Work out the finished part from the listing and answer in its coordinate system (mm). A direction names the side the tool comes from. Coordinates: 2 decimals unless noted, no trailing zeros. Write each loop counter-clockwise with the first axis right and the second up, starting at its lowest first coordinate (ties: lowest second). Pieces come first, ordered by that corner, then holes. Notation, with made-up numbers: (-32.5, 57.5) - (21.5, 57.5) arc R10 ccw to (21.5, 73.5) - close; hole circle Ø11 at (4.25, -35). An arc over 180 degrees is marked (long way). Use a Markdown table: item, result. Add a question column.
(1) The part is cut by section D-D, the plane y = 15. Give the vertices of the cut face in (x, z).
(2) Find the intervals of material crossed by line 1 (Z direction, x = 32, y = 9.5); line 2 (X direction, y = 4.5, z = 38.05); line 3 (Y direction, x = 12.25, z = 2.25), in increasing order. Write a range as from..to.
(3) A tool of negligible diameter and unlimited length cuts with its end or side. For faces 1 (the face through (21.405, 20.021, 2.535)), 2 (the face through (20, 13, 5)), 3 (the face through (29.405, 20.021, 37.465)), from which of +Z, -Z, +X, -X, +Y, -Y can it reach the whole face along a straight path? Write none if from no direction.
(4) The part is cut by section A-A, the plane x = 16. Give the vertices of the cut face in (y, z), then the cut area to 3 significant figures.
(5) For a pull along Y with two mould halves and no side action, classify faces 4 (the face through (12.09, 13.74, 37.47)), 5 (the face through (20, 25, 20)), 6 (the face through (20, 12, 22.5)), 7 (the face through (29.405, 20.021, 2.535)) as released by +Y, released by -Y, zero draft, split by the parting line, or undercut.
(6) The part is cut by section B-B, the plane y = 11.75. State how many separate pieces and enclosed holes the cut face has, then the cut area to 3 significant figures.
(7) The part is cut by section C-C, the plane z = 27. Give the vertices of the cut face in (x, y).
(8) Given pin 1 Ø1.5 at (x, y) = (20.25, 4.5) entering from +Z; pin 2 Ø1 at (x, y) = (29, 5) entering from -Z; pin 3 Ø1.5 at (x, y) = (12.25, 4.5) entering from -Z, each flat-ended and moving along its own axis, determine where each tip first touches the part or whether it passes through.
from build123d import *

# Parameters (mm, degrees)
SKETCH1_W               = 40.5
SKETCH1_H               = 25
BOSS_EXTRUDE1_DEPTH     = 40
CUT_EXTRUDE1_START      = -5
SKETCH2_W               = 26.5
SKETCH2_H               = 25
CUT_EXTRUDE1_DEPTH      = 30
FILLET1_R               = 1
SKETCH3_R               = 1.25
CUT_EXTRUDE2_DEPTH      = 35
CUT_EXTRUDE2_DEPTH_BACK = 5
FILLET2_R               = 1
SKETCH6_W               = 5
SKETCH6_H               = 25
BOSS_EXTRUDE3_DEPTH     = 40.5


with BuildPart() as part:
    # Sketch1 → Boss-Extrude1 (new body)
    with BuildSketch(Plane.XY):
        with Locations((20.25, 12.5)):
            Rectangle(SKETCH1_W, SKETCH1_H)
    extrude(amount=BOSS_EXTRUDE1_DEPTH)

    # Sketch2 → Cut-Extrude1 (cut)
    with BuildSketch(Plane.XY.offset(40).offset(CUT_EXTRUDE1_START)):
        with Locations((20.25, 12.5)):
            Rectangle(SKETCH2_W, SKETCH2_H)
    extrude(amount=-CUT_EXTRUDE1_DEPTH, mode=Mode.SUBTRACT)

    # Fillet1
    fillet1_edges = [part.edges().sort_by_distance(p)[0] for p in [
        (40.5, 12.5, 0),
        (0, 12.5, 0),
    ]]
    fillet(fillet1_edges, radius=FILLET1_R)

    # Sketch3 → Cut-Extrude2 (cut, two sides)
    with BuildSketch(Plane.XY.offset(5)) as cut_extrude2_sk:
        with Locations((12.25, 4.5)):
            Circle(SKETCH3_R)
        with Locations((20.25, 4.5)):
            Circle(SKETCH3_R)
        with Locations((12.25, 12.5)):
            Circle(SKETCH3_R)
        with Locations((12.25, 20.5)):
            Circle(SKETCH3_R)
        with Locations((20.25, 20.5)):
            Circle(SKETCH3_R)
        with Locations((28.25, 4.5)):
            Circle(SKETCH3_R)
        with Locations((28.25, 12.5)):
            Circle(SKETCH3_R)
        with Locations((28.25, 20.5)):
            Circle(SKETCH3_R)
    extrude(amount=CUT_EXTRUDE2_DEPTH, mode=Mode.SUBTRACT)
    extrude(cut_extrude2_sk.sketch, amount=-CUT_EXTRUDE2_DEPTH_BACK, mode=Mode.SUBTRACT)

    # Fillet2
    fillet2_edges = [part.edges().sort_by_distance(p)[0] for p in [
        (40.5, 12.5, 40),
        (0, 12.5, 40),
    ]]
    fillet(fillet2_edges, radius=FILLET2_R)

    # Sketch6 → Boss-Extrude3 (add)
    with BuildSketch(Plane(origin=(40.5, 0, 0), x_dir=(0, 0, -1), z_dir=(1, 0, 0))):
        with Locations((-20, 12.5)):
            Rectangle(SKETCH6_W, SKETCH6_H)
    extrude(amount=-BOSS_EXTRUDE3_DEPTH)


solid = part.part
Model answer:
| question | item | result |
|---|---|---|
| 1 | outline | (0, 1) arc R1 ccw to (1, 0) - (39.5, 0) arc R1 ccw to (40.5, 1) - (40.5, 39) arc R1 ccw to (39.5, 40) - (1, 40) arc R1 ccw to (0, 39) - close; hole (7, 5) - (33.5, 5) - (33.5, 17.5) - (7, 17.5) - close; hole (7, 22.5) - (33.5, 22.5) - (33.5, 35) - (7, 35) - close |
| 2 | line 1 | 0..5, 17.5..22.5, 35..40 |
| 2 | line 2 | 0..11, 13.5..19, 21.5..27, 29.5..40.5 |
| 2 | line 3 | 0..3.25, 5.75..11.25, 13.75..19.25, 21.75..25 |
| 3 | face 1 | -Z |
| 3 | face 2 | +Y, -Y |
| 3 | face 3 | +Z |
| 4 | outline | (0, 0) - (25, 0) - (25, 5) - (0, 5) - close; (0, 17.5) - (25, 17.5) - (25, 22.5) - (0, 22.5) - close; (0, 35) - (25, 35) - (25, 40) - (0, 40) - close |
| 4 | area | 375 mm^2 |
| 5 | face 4 | undercut |
| 5 | face 5 | released by +Y |
| 5 | face 6 | zero draft |
| 5 | face 7 | undercut |
| 6 | separate pieces | 3 |
| 6 | enclosed holes | 0 |
| 6 | area | 917 mm^2 |
| 7 | outline | (0, 0) - (7, 0) - (7, 25) - (0, 25) - close; (33.5, 0) - (40.5, 0) - (40.5, 25) - (33.5, 25) - close |
| 8 | pin 1 | z = 22.5 |
| 8 | pin 2 | z = 0 |
| 8 | pin 3 | z = 17.5 |
